The figure shows three views and two pictorial views of one solid part (mm, origin at its lowest corner). Answer the questions. A direction names the side the tool comes from. Round coordinates to 2 decimals unless told otherwise and drop trailing zeros. Write each loop counter-clockwise with the first axis right and the second up, starting at its lowest first coordinate (ties: lowest second). Pieces come first, ordered by that corner, then holes. Notation, with made-up numbers: M -9,21.5 L 47,21.5 A31 cw 47,50.5 Z; hole C 71.5,0 d7. An arc over 180 degrees is marked long. Use one line per item in the form item = value. Start each with the question number.
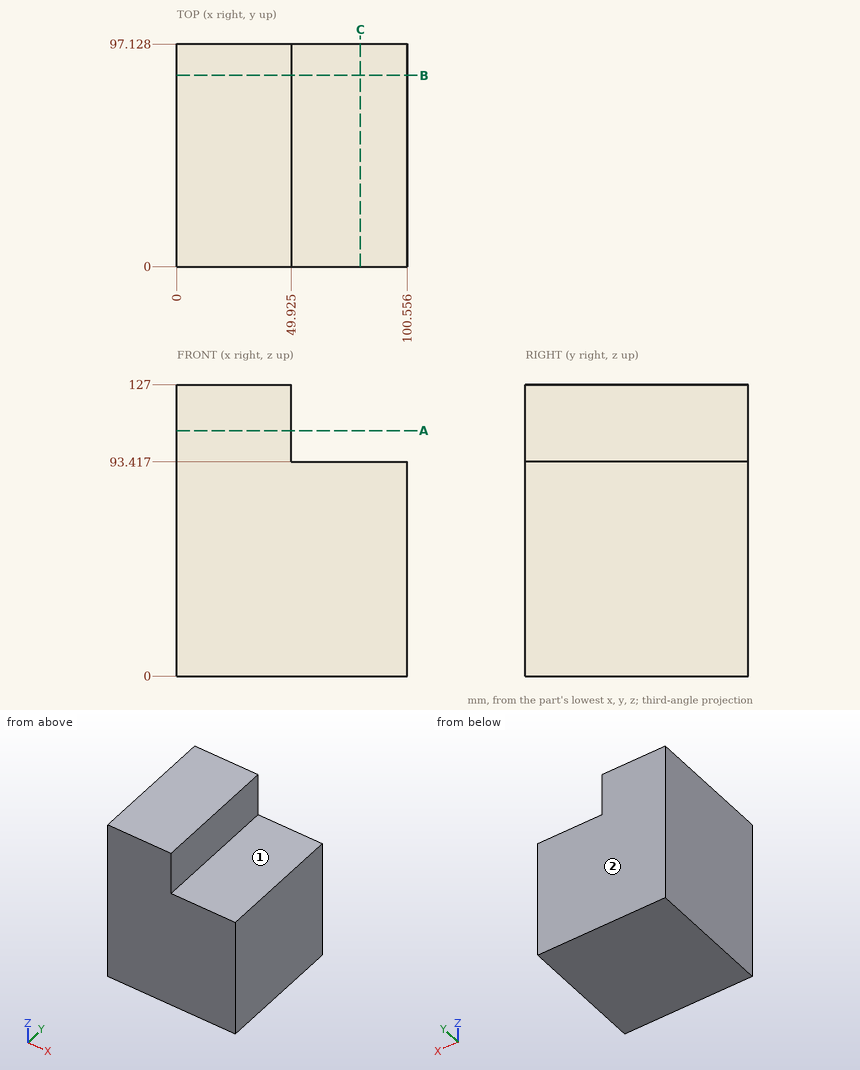
Q1. A tool of negligible diameter and unlimited length cuts with its end or side. For the marked faces 1 and 2, from which of +Z, -Z, +X, -X, +Y, -Y can it reach the whole face along a straight path? Write none if from no direction.
Q2. Straight lines are drawn through the part: line 1 (Z direction, x = 96.5, y = 12); line 2 (X direction, y = 63.5, z = 106) (1 decimal). For each, find the intervals that lie inside material, in ascending order. Write a range as [from, to].
Q3. Find section A-A on z = 107. Write down the section's boundary in (x, y) (1 decimal).
Q4. Find section C-C on x = 80. Write down the section's boundary in (y, z), and give its area (3 significant figures).
Q5. Find section B-B on y = 83.5. Write down the section's boundary in (x, z) (1 decimal), and give its area (3 significant figures).
Q6. Each of these flat-tipped pins is pushed along its axis until it touches: pin 1 Ø1.5 at (y, z) = (80, 78.5) entering from -X; pin 2 Ø17 at (y, z) = (68, 115) entering from +X (3 decimals). Where does it stop, or does it pass through?
Response:
q1.face_1 = +Z, +X, +Y, -Y
q1.face_2 = +Z, -Z, +X, -X, +Y
q2.line_1 = [0, 93.42]
q2.line_2 = [0, 49.9]
q3.outline = M 0,0 L 49.9,0 L 49.9,97.1 L 0,97.1 Z
q4.outline = M 0,0 L 97.13,0 L 97.13,93.42 L 0,93.42 Z
q4.area = 9,070 mm²
q5.outline = M 0,0 L 100.6,0 L 100.6,93.4 L 49.9,93.4 L 49.9,127 L 0,127 Z
q5.area = 11,100 mm²
q6.pin_1 = 0
q6.pin_2 = 49.925
